Autodesk Inventor part; units mm, degrees
ref_plane "YZ Plane" through (0, 0, 0) normal (1, 0, 0) x (0, 1, 0)
ref_plane "XZ Plane" through (0, 0, 0) normal (0, 1, 0) x (-1, 0, 0)
ref_plane "XY Plane" through (0, 0, 0) normal (0, 0, 1) x (1, 0, 0)
sketch "Sketch1" plane through (0, 0, 0) normal (1, 0, 0) x (0, 1, 0)
  circle A0 centre (0, 0) radius 4
  circle A1 centre (0, 0) radius 6
  dimension "d0" = 8
  dimension "d1" = 12
extrude "Extrusion1" add sketch "Sketch1" along normal blind 25
sketch "Sketch2" plane through (25, 0, 0) normal (1, 0, 0) x (0, 0, -1)
  circle A0 centre (0, 0) radius 4
extrude "Extrusion2" add sketch "Sketch2" along normal blind 740
sketch "Sketch3" plane through (25, 0, 0) normal (1, 0, 0) x (0, 0, -1)
  circle A0 centre (0, 0) radius 4
  circle A1 centre (0, 0) radius 6.0091
extrude "Extrusion3" add sketch "Sketch3" along normal blind 10
sketch "Sketch4" plane through (0, 0, 0) normal (0, 0, 1) x (1, 0, 0)
  line L0 (25, 4) -> (25, -4)
  line L1 (25, 0) -> (15, 0)
  circle A0 centre (15, 0) radius 2
  point P0 (0, 0)
  dimension "d9" = 10
  dimension "d10" = 4
extrude "Extrusion4" cut sketch "Sketch4" along normal blind 740
thread "Thread1"
sketch "Sketch5" plane through (0, 0, 0) normal (0, 0, 1) x (1, 0, 0)
  line L0 (765, -4) -> (765, 4)
  line L1 (765, 0) -> (755, 0)
  circle A0 centre (755, -0.2044) radius 2
  point P0 (0, 0)
  dimension "d15" = 10
  dimension "d16" = 4
extrude "Extrusion5" cut sketch "Sketch5" along normal blind 60
chamfer "Chamfer1" distance 0.5 angle 45 1 edges at (753.0009, -0.2632, 3.9913)
properties part number "700_achse"
Part model, mm, in its own coordinate system. A direction names the side the tool comes from. Coordinates: 2 decimals unless noted, no trailing zeros. Write each loop counter-clockwise with the first axis right and the second up, starting at its lowest first coordinate (ties: lowest second). Pieces come first, ordered by that corner, then holes.
Item 1: Pin check, flat tips, straight feed: pin 1 (6.5 mm diameter, centred on y = 0, z = -1, fed in from -X); pin 2 (6 mm diameter, centred on x = 531, z = 1, fed in from +Y); pin 3 (2 mm diameter, centred on x = 595, y = -4.5, fed in from -Z); pin 4 (3.5 mm diameter, centred on x = 755, y = -0.2, fed in from -Z). Stop position of each tip, or through.
Item 2: Probe line 1 (X direction, y = -0.75, z = 3.5); line 2 (Z direction, x = 8.75, y = 0); line 3 (Y direction, x = 15, z = 4.45). List the from-to ranges inside material, lowest first.
Item 3: Slice it at A-A (x = 262.5). Write the cut outline in (y, z).
Item 4: Which spindle directions (+Z, -Z, +X, -X, +Y, -Y) get a long thin tool onto all of the face, cutting with end or side? Do faces 1 (the face through (35, -3.92, 1.42)), 2 (the face through (0, -1.42, -3.92)). Say none if no direction does.
Results found:
1. pin 1: stops at x = 0
1. pin 2: stops at y = 4
1. pin 3: stops at z = -1.94
1. pin 4: stops at z = -4
2. line 1: x = 25 to 752.99, 757.01 to 765
2. line 2: z = -6 to -4, 4 to 6
2. line 3: y = -4.02 to -2, 2 to 4.02
3. outline: circle Ø8 at (0, 0)
4. face 1: +X
4. face 2: +Z, -Z, -X, +Y, -Y
